Verification items for the finished model (mm, model axes). A direction names the side the tool comes from. Give positions to 0.01 mm unless a question says otherwise; leave off trailing zeros. Order: outer loops, then holes, each group sorted by start corner. A loop starts at its lowest first (then second) coordinate and runs counter-clockwise, first axis right, second up.
from build123d import *

# Parameters (mm, degrees)
SKETCH_1_W      = 23.8
SKETCH_1_H      = 10
SKETCH_1_R      = 2.25
SKETCH_1_H_2    = 16.8
SKETCH_1_W_2    = 21.8
SKETCH_1_H_3    = 14.8
EXTRUDE_1_DEPTH = 2
EXTRUDE_START   = 2
SKETCH_1_3_W    = 23.8
SKETCH_1_3_H    = 16.8
SKETCH_1_3_W_2  = 21.8
SKETCH_1_3_H_2  = 14.8
EXTRUDE_2_DEPTH = 2


with BuildPart() as part:
    # 草图1 → 凸台-拉伸1 (new body)
    # profile 1 of 3: a face of its own
    with BuildSketch(Plane(origin=(0, 0, 0), x_dir=(1, 0, 0), z_dir=(0, 1, 0))):
        with Locations((0, 13.4)):
            Rectangle(SKETCH_1_W, SKETCH_1_H)
        with Locations(Location((0, 13.4, 0), (0, 0, 270))):
            Circle(SKETCH_1_R, mode=Mode.SUBTRACT)
        with Locations(Location((-8, 13.4, 0), (0, 0, 270))):
            Circle(SKETCH_1_R, mode=Mode.SUBTRACT)
        with Locations(Location((8, 13.4, 0), (0, 0, 270))):
            Circle(SKETCH_1_R, mode=Mode.SUBTRACT)
    # profile 2 of 3: a face of its own
    with BuildSketch(Plane(origin=(0, 0, 0), x_dir=(1, 0, 0), z_dir=(0, 1, 0))):
        Rectangle(SKETCH_1_W, SKETCH_1_H_2)
        Rectangle(SKETCH_1_W_2, SKETCH_1_H_3, mode=Mode.SUBTRACT)
    # profile 3 of 3: a face of its own
    with BuildSketch(Plane(origin=(0, 0, 0), x_dir=(1, 0, 0), z_dir=(0, 1, 0))):
        Rectangle(SKETCH_1_W_2, SKETCH_1_H_3)
    extrude(amount=EXTRUDE_1_DEPTH)

    # 草图1<3> → 凸台-拉伸2 (add)
    with BuildSketch(Plane(origin=(0, 0, 0), x_dir=(1, 0, 0), z_dir=(0, 1, 0)).offset(EXTRUDE_START)):
        Rectangle(SKETCH_1_3_W, SKETCH_1_3_H)
        Rectangle(SKETCH_1_3_W_2, SKETCH_1_3_H_2, mode=Mode.SUBTRACT)
    extrude(amount=EXTRUDE_2_DEPTH)


solid = part.part
(1) Set-up check for faces 4 (the flat face through (0, 2, 8.4)), 5 (the flat face through (0, 2, -16)), 6 (the flat face through (0, 2, 0)): record each of +Z, -Z, +X, -X, +Y, -Y from which the full face is reachable in a straight line by a thin tool's end or side.
Solved:
face 4: +Z, +X, -X, +Y, -Y
face 5: -Z, +X, -X, +Y
face 6: +Y
(2) Section check D-D, the plane z = -2.25. Enter the section's corners in (x, y).
Solved:
outline: (-11.9, 0) - (11.9, 0) - (11.9, 4) - (10.9, 4) - (10.9, 2) - (-10.9, 2) - (-10.9, 4) - (-11.9, 4) - close
(3) Section check A-A, the plane z = -13.4. Enter the section's corners in (x, y).
Solved:
outline: (-11.9, 0) - (-10.25, 0) - (-10.25, 2) - (-11.9, 2) - close; (-5.75, 0) - (-2.25, 0) - (-2.25, 2) - (-5.75, 2) - close; (2.25, 0) - (5.75, 0) - (5.75, 2) - (2.25, 2) - close; (10.25, 0) - (11.9, 0) - (11.9, 2) - (10.25, 2) - close
(4) Section check B-B, the plane y = 0.65. Enter the section's corners in (x, z).
Solved:
outline: (-11.9, -18.4) - (11.9, -18.4) - (11.9, 8.4) - (-11.9, 8.4) - close; hole circle Ø4.5 at (-8, -13.4); hole circle Ø4.5 at (0, -13.4); hole circle Ø4.5 at (8, -13.4)
(5) Go/stop test with flat-tipped pins: pin 1 (2 mm diameter, centred on x = 6, z = -13, fed in from +Y); pin 2 (0.6 mm diameter, centred on x = 1.5, y = 3, fed in from -Z); pin 3 (4 mm diameter, centred on x = -8, z = -13.4, fed in from -Y). Record where each tip stops, or that it passes through.
Solved:
pin 1: stops at y = 2
pin 2: stops at z = -8.4
pin 3: passes through
(6) Release check for a two-part mould opening along Z. For faces 1 (the flat face through (0, 3, -8.4)), 2 (the flat face through (11.9, 2, -2)), 3 (the cylindrical face through (0.676, 0.986, -11.254)) record: pulls with the +Z half, pulls with the -Z half, needs draft (parallel to the pull), parting line crosses it, or undercut.
Solved:
face 1: pulls with the -Z half
face 2: needs draft
face 3: undercut
(7) Section check C-C, the plane x = -8. Enter the section's corners in (y, z).
Solved:
outline: (0, -18.4) - (2, -18.4) - (2, -15.65) - (0, -15.65) - close; (0, -11.15) - (2, -11.15) - (2, -8.4) - (4, -8.4) - (4, -7.4) - (2, -7.4) - (2, 7.4) - (4, 7.4) - (4, 8.4) - (0, 8.4) - close
(8) Scan lines: line 1 (X direction, y = 0.8, z = -13.4); line 2 (X direction, y = 3.5, z = -3); line 3 (Z direction, x = -7, y = 3.85). Record each from-to range of solid material in increasing order.
Solved:
line 1: x = -11.9 to -10.25, -5.75 to -2.25, 2.25 to 5.75, 10.25 to 11.9
line 2: x = -11.9 to -10.9, 10.9 to 11.9
line 3: z = -8.4 to -7.4, 7.4 to 8.4
